Geometry: see drawing. Coordinates: mm, zero at the bounding-box minimum. A direction names the side the tool comes from. Give positions to 0.01 mm unless a question says otherwise; leave off trailing zeros. Write each loop counter-clockwise with the first axis right and the second up, starting at its lowest first coordinate (ties: lowest second). Pieces come first, ordered by that corner, then holes. Notation, with made-up numbers: (3, -12) -> (30, -12) arc R23 ccw to (30, 7) -> close; hole circle Ø8 at (45, 56.5). An arc over 180 degrees is marked (long way). Answer as a JSON object with one key per item and string values. Group by question number.
Item 1: First-contact query: pin 1 Ø12 at (y, z) = (47, 38.5) entering from +X; pin 2 Ø12 at (y, z) = (72.5, 58.5) entering from -X; pin 3 Ø3 at (x, z) = (65.4, 11.9) entering from +Y; pin 4 Ø4 at (x, z) = (55.5, 73.5) entering from +Y. Flat tips, straight axial feed; report the tip coordinate or a pass-through.
Item 2: Access query for the marked faces 4, 5 and 6. Directions: +Z, -Z, +X, -X, +Y, -Y. A direction counts if a zero-diameter tool reaches every point of the face in a straight line with its end or side. Return the directions, or none.
Item 3: Section query D-D on x = 65.4. Return the cut outline in (y, z) (3 decimals), plus the area to 3 significant figures.
Item 4: Ray query, probe 1 along X at (y, z) = (3, 11.9) (3 decimals); probe 2 along Z at (x, y) = (14.6, 5.5) (3 decimals); probe 3 along Y at (x, z) = (44.25, 50). Return the intervals inside material, ascending. Write a range as from..to.
Item 5: Section query A-A on y = 103.69. Return the cut outline in (x, z), plus the area to 3 significant figures.
Item 6: Section query C-C on z = 88.1. Return the cut outline in (x, y) (3 decimals).
Item 7: Pull-direction query (Y, two-part tool) for the marked faces 1, 2 and 3; classes: pulls with the +Y half, pulls with the -Y half, needs draft (parallel to the pull), parting line crosses it, or undercut.
Item 8: Section query B-B on z = 38. Return the cut outline in (x, y).
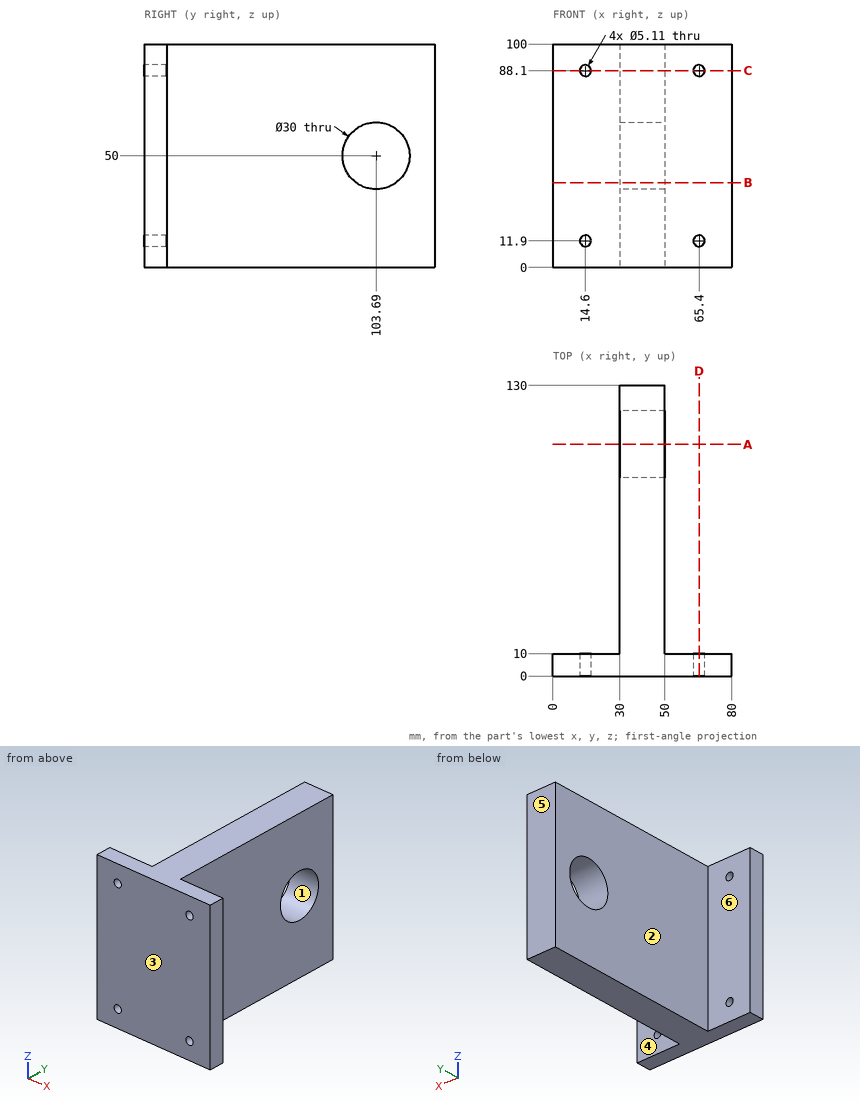
Worked answers:
{
 "1": {"pin 1": "x = 50", "pin 2": "x = 30", "pin 3": "through", "pin 4": "y = 10"},
 "2": {"face 4": "+Z, -Z, +X, +Y", "face 5": "+Z, -Z, +X, -X, +Y", "face 6": "+Z, -Z, -X, +Y"},
 "3": {"outline": "(0, 0) -> (10, 0) -> (10, 9.345) -> (0, 9.345) -> close; (0, 14.455) -> (10, 14.455) -> (10, 85.545) -> (0, 85.545) -> close; (0, 90.655) -> (10, 90.655) -> (10, 100) -> (0, 100) -> close", "area": "898 mm^2"},
 "4": {"probe 1": "0..12.045, 17.155..62.845, 67.955..80", "probe 2": "0..9.345, 14.455..85.545, 90.655..100", "probe 3": "0..88.69, 118.69..130"},
 "5": {"outline": "(30, 0) -> (50, 0) -> (50, 35) -> (30, 35) -> close; (30, 65) -> (50, 65) -> (50, 100) -> (30, 100) -> close", "area": "1,400 mm^2"},
 "6": {"outline": "(0, 0) -> (12.045, 0) -> (12.045, 10) -> (0, 10) -> close; (17.155, 0) -> (62.845, 0) -> (62.845, 10) -> (50, 10) -> (50, 130) -> (30, 130) -> (30, 10) -> (17.155, 10) -> close; (67.955, 0) -> (80, 0) -> (80, 10) -> (67.955, 10) -> close"},
 "7": {"face 1": "undercut", "face 2": "needs draft", "face 3": "pulls with the -Y half"},
 "8": {"outline": "(0, 0) -> (80, 0) -> (80, 10) -> (50, 10) -> (50, 94.69) -> (30, 94.69) -> (30, 10) -> (0, 10) -> close; (30, 112.69) -> (50, 112.69) -> (50, 130) -> (30, 130) -> close"}
}
